Verification items for the finished model (mm, model axes). Coordinates: 2 decimals unless noted, no trailing zeros. Loops run counter-clockwise (first coordinate to the right, second up) from the corner with the lowest first, then second, coordinate; pieces in that order, holes last. Notation, with made-up numbers: (49, 4) -> (92, 4) arc R22 ccw to (92, 18) -> close; hole circle Ø2 at (-11, 43). An arc over 180 degrees is marked (long way). Answer as a JSON object with one key per item and string values. Group by question number.
Q1. Cross-section at B-B on x = 109.5. Record the boundary of the cut face in (y, z), and give its area (3 significant figures).
Q2. Scan lines: L1, parallel to Y at x = 100, z = 9.3; L2, parallel to Y at x = 0, z = 7; L3, parallel to X at y = 30, z = 5. Record each from-to range of solid material in increasing order.
Q3. Cross-section at C-C on z = 4.75. Give the number of separate pieces and of enclosed holes in the cut face, and give its area (3 significant figures).
Q4. Cross-section at A-A on y = 0. Record the boundary of the cut face in (x, z).
Q5. Gauge pin test, flat ends, axial feed: pin 1 Ø5 at (x, y) = (131.5, -96) entering from -Z; pin 2 Ø2.5 at (x, y) = (125.98, 15) entering from +Z; pin 3 Ø3.5 at (x, y) = (100, 30) entering from +Z. Record the tip position at first contact, or that the pin passes through.
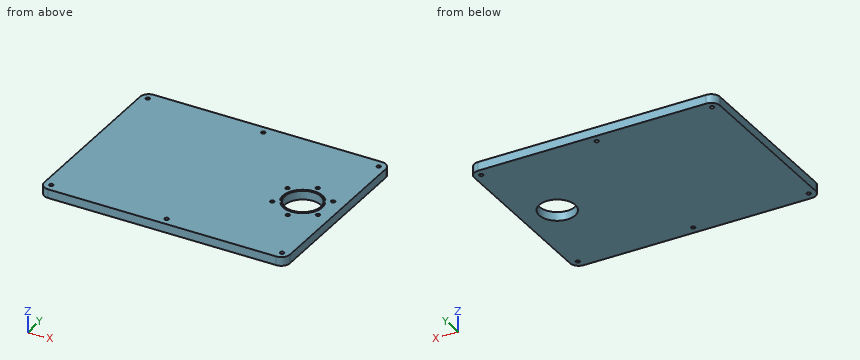
```python
from build123d import *

# Parameters (mm, degrees)
F0_W     = 280
F0_H     = 210
F1_DEPTH = 10
F2_R     = 20.5
F3_DEPTH = 10
F5_R     = 10
F7_D     = 4.5
F8_D     = 4.5
F8_DEPTH = 8
F8_TIP   = 1.3519363928
F2_R_2   = 22.65
F2_R_3   = 21.35
F9_DEPTH = 1


with BuildPart() as f1:
    # F0 (on Top) → F1 (new body)
    with BuildSketch(Plane.XY):
        Rectangle(F0_W, F0_H)
    extrude(amount=F1_DEPTH)


with BuildPart() as f3:
    # F2 (on face) → F3 (new body)
    with BuildSketch(Plane.XY.offset(10)):
        with Locations((100, 0)):
            Circle(F2_R)
    extrude(amount=-F3_DEPTH)


with BuildPart() as f1_1:
    add(f1.part)

    # F4: cut F3
    add(f3.part, mode=Mode.SUBTRACT)

    # F5
    f5_edges = [f1_1.edges().sort_by_distance(p)[0] for p in [
        (-140, 105, 5),
        (140, 105, 5),
        (140, -105, 5),
        (-140, -105, 5),
    ]]
    fillet(f5_edges, radius=F5_R)

    # F7 (through all)
    with Locations(Plane.XY.offset(10)):
        with Locations((-131.5, 96), (0, 96), (131.5, 96), (131.5, -96), (0, -96), (-131.5, -96)):
            Hole(F7_D / 2)

    # F8
    with Locations(Plane.XY.offset(10)):
        with Locations((100, 30), (125.9807621135, 15), (125.9807621135, -15), (100, -30), (74.0192378865, -15), (74.0192378865, 15)):
            Hole(F8_D / 2, depth=F8_DEPTH)
            with Locations((0, 0, -(F8_DEPTH + F8_TIP / 2))):  # 118° drill point
                Cone(0, F8_D / 2, F8_TIP, mode=Mode.SUBTRACT)


with BuildPart() as f9:
    # F2 (on face) → F9 (new body)
    with BuildSketch(Plane.XY.offset(10)):
        with Locations((100, 0)):
            Circle(F2_R_2)
        with Locations((100, 0)):
            Circle(F2_R_3, mode=Mode.SUBTRACT)
    extrude(amount=-F9_DEPTH)


with BuildPart() as f1_2:
    add(f1_1.part)

    # F10: cut F9
    add(f9.part, mode=Mode.SUBTRACT)


solid = f1_2.part
```
Computed values:
{
 "1": {"outline": "(-105, 0) -> (-18.17, 0) -> (-18.17, 10) -> (-19.12, 10) -> (-19.12, 9) -> (-20.56, 9) -> (-20.56, 10) -> (-105, 10) -> close; (18.17, 0) -> (105, 0) -> (105, 10) -> (20.56, 10) -> (20.56, 9) -> (19.12, 9) -> (19.12, 10) -> (18.17, 10) -> close", "area": "1,730 mm²"},
 "2": {"L1": "y = -105 to -32.25, -27.75 to -22.65, -21.35 to -20.5, 20.5 to 21.35, 22.65 to 27.75, 32.25 to 105", "L2": "y = -105 to -98.25, -93.75 to 93.75, 98.25 to 105", "L3": "x = -140 to 97.75, 102.25 to 140"},
 "3": {"separate pieces": "1", "enclosed holes": "13", "area": "57,200 mm²"},
 "4": {"outline": "(-140, 0) -> (79.5, 0) -> (79.5, 10) -> (78.65, 10) -> (78.65, 9) -> (77.35, 9) -> (77.35, 10) -> (-140, 10) -> close; (120.5, 0) -> (140, 0) -> (140, 10) -> (122.65, 10) -> (122.65, 9) -> (121.35, 9) -> (121.35, 10) -> (120.5, 10) -> close"},
 "5": {"pin 1": "stops at z = 0", "pin 2": "stops at z = 1.4", "pin 3": "stops at z = 1.7"}
}
